Build history of the part. All positions in model axes, mm. Face numbers are marked on the shaded views. A direction names the side the tool comes from. Round coordinates to 2 decimals unless told otherwise and drop trailing zeros. Write each loop counter-clockwise with the first axis right and the second up, starting at its lowest first coordinate (ties: lowest second). Pieces come first, ordered by that corner, then holes. Notation, with made-up numbers: (9.5, -36.5) -> (32.5, -36.5) arc R21 cw to (32.5, -3.5) -> close; hole circle Ø5 at (79.25, -25.5). An arc over 180 degrees is marked (long way). Answer in a Markdown table with one row per item. Add a question column.
from build123d import *

# Parameters (mm, degrees)
F0_R      = 27.5
F2_DEPTH  = 40
F4_W      = 100
F4_H      = 100
F5_DEPTH  = 10
F3_R      = 20
F6_DEPTH  = 40.001
F1_R      = 23.5
F7_DEPTH  = 40.001
F10_R     = 2
F11_R     = 0.5
F8_R      = 8
F9_R      = 4
F12_DEPTH = 15


with BuildPart() as f2:
    # F0 (on Top) → F2 (new body, symmetric)
    with BuildSketch(Plane.XY):
        Circle(F0_R)
    extrude(amount=F2_DEPTH, both=True)

    # F4 (on Top) → F5 (join, symmetric)
    with BuildSketch(Plane.XY):
        Rectangle(F4_W, F4_H)
    extrude(amount=F5_DEPTH, both=True)

    # F3 (on Top) → F6 (cut, through all)
    with BuildSketch(Plane.XY):
        Circle(F3_R)
    extrude(amount=-F6_DEPTH, mode=Mode.SUBTRACT)

    # F1 (on Top) → F7 (cut, through all)
    with BuildSketch(Plane.XY):
        Circle(F1_R)
    extrude(amount=F7_DEPTH, mode=Mode.SUBTRACT)

    # F10
    f10_edges = [f2.edges().sort_by_distance(p)[0] for p in [
        (-27.5, 0, 10),
        (-27.5, 0, -10),
    ]]
    fillet(f10_edges, radius=F10_R)

    # F11
    f11_edges = [f2.edges().sort_by_distance(p)[0] for p in [
        (-27.5, 0, -40),
        (-27.5, 0, 40),
    ]]
    fillet(f11_edges, radius=F11_R)

    # F8 (on Top) + F9 (on Top) → F12 (cut, symmetric)
    with BuildSketch(Plane.XY):
        with Locations((0, -38)):
            Circle(F8_R)
    with BuildSketch(Plane.XY):
        with Locations((0, 40)):
            Circle(F9_R)
    extrude(amount=F12_DEPTH, both=True, mode=Mode.SUBTRACT)


solid = f2.part
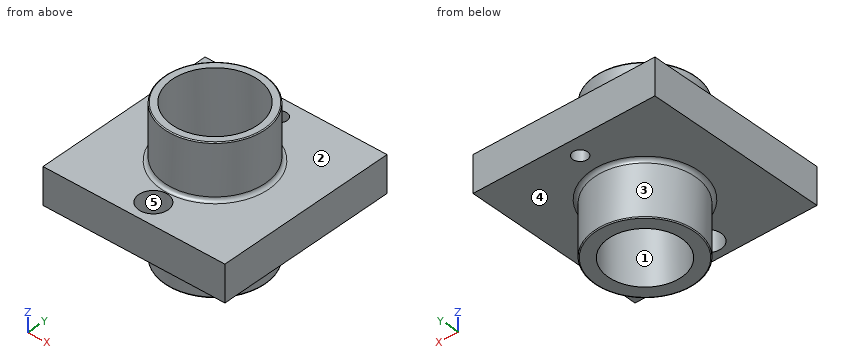
(1) Saw through at D-D (x = 0). Count the separate pieces of the cut face and the enclosed holes in it, plus the area to 3 significant figures.
(2) Which spindle directions (+Z, -Z, +X, -X, +Y, -Y) get a long thin tool onto all of the face, cutting with end or side? Do the marked faces 1 and 2. Say none if no direction does.
(3) Mould opens along Y. For the marked faces 3, 4 and 5 say: pulls with the +Y half, pulls with the -Y half, needs draft (parallel to the pull), parting line crosses it, or undercut.
(4) Drop flat-ended pins along their axis: P1, Ø12, axis at x = -25, z = 28.5, coming from the +Y side; P2, Ø10, axis at x = 2, z = -28, coming from the -Y side; P3, Ø1, axis at y = 20, z = 31.5, coming from the +X side. Give the stop position or say it passes through.
(5) Probe line 1 along Y through (x, z) = (0, 4); line 2 along Y through (x, z) = (0, -21); line 3 along Z through (x, y) = (39.5, -19). List the from-to ranges inside material, lowest first.
(6) Saw through at A-A (y = 40). List the corners of the cut face in (x, z), plus the area to 3 significant figures.
(7) Saw through at C-C (x = 34). List the corners of the cut face in (y, z).
(8) Saw through at B-B (y = 0). List the corners of the cut face in (x, z).
Answer sheet:
| question | item | result |
|---|---|---|
| 1 | separate pieces | 4 |
| 1 | enclosed holes | 0 |
| 1 | area | 1,340 mm² |
| 2 | face 1 | +Z, -Z |
| 2 | face 2 | +Z |
| 3 | face 3 | parting line crosses it |
| 3 | face 4 | needs draft |
| 3 | face 5 | undercut |
| 4 | P1 | stops at y = 19.88 |
| 4 | P2 | stops at y = -27.5 |
| 4 | P3 | stops at x = 19.39 |
| 5 | line 1 | y = -50 to -46, -30 to -23.5, 23.5 to 36, 44 to 50 |
| 5 | line 2 | y = -27.5 to -20, 20 to 27.5 |
| 5 | line 3 | z = -10 to 10 |
| 6 | outline | (-50, -10) -> (-4, -10) -> (-4, 10) -> (-50, 10) -> close; (4, -10) -> (50, -10) -> (50, 10) -> (4, 10) -> close |
| 6 | area | 1,840 mm² |
| 7 | outline | (-50, -10) -> (50, -10) -> (50, 10) -> (-50, 10) -> close |
| 8 | outline | (-50, -10) -> (-29.5, -10) arc R2 cw to (-27.5, -12) -> (-27.5, -39.5) arc R0.5 ccw to (-27, -40) -> (-20, -40) -> (-20, 0) -> (-23.5, 0) -> (-23.5, 40) -> (-27, 40) arc R0.5 ccw to (-27.5, 39.5) -> (-27.5, 12) arc R2 cw to (-29.5, 10) -> (-50, 10) -> close; (20, -40) -> (27, -40) arc R0.5 ccw to (27.5, -39.5) -> (27.5, -12) arc R2 cw to (29.5, -10) -> (50, -10) -> (50, 10) -> (29.5, 10) arc R2 cw to (27.5, 12) -> (27.5, 39.5) arc R0.5 ccw to (27, 40) -> (23.5, 40) -> (23.5, 0) -> (20, 0) -> close |
